```python
from build123d import *

# Parameters (mm, degrees)
SKETCH_1_W      = 150
SKETCH_1_H      = 20
SKETCH_1_W_2    = 25
SKETCH_1_H_2    = 3
EXTRUDE_1_DEPTH = 3


with BuildPart() as part:
    # 草图1 → 凸台-拉伸1 (new body)
    with BuildSketch(Plane(origin=(0, 0, 0), x_dir=(1, 0, 0), z_dir=(0, 1, 0))):
        Rectangle(SKETCH_1_W, SKETCH_1_H)
        with Locations((-60, 11.5)):
            Rectangle(SKETCH_1_W_2, SKETCH_1_H_2)
        with Locations((-60, -11.5)):
            Rectangle(SKETCH_1_W_2, SKETCH_1_H_2)
        with Locations((0, -11.5)):
            Rectangle(SKETCH_1_W_2, SKETCH_1_H_2)
        with Locations((0, 11.5)):
            Rectangle(SKETCH_1_W_2, SKETCH_1_H_2)
        with Locations((60, 11.5)):
            Rectangle(SKETCH_1_W_2, SKETCH_1_H_2)
        with Locations((60, -11.5)):
            Rectangle(SKETCH_1_W_2, SKETCH_1_H_2)
    extrude(amount=EXTRUDE_1_DEPTH)


solid = part.part
```
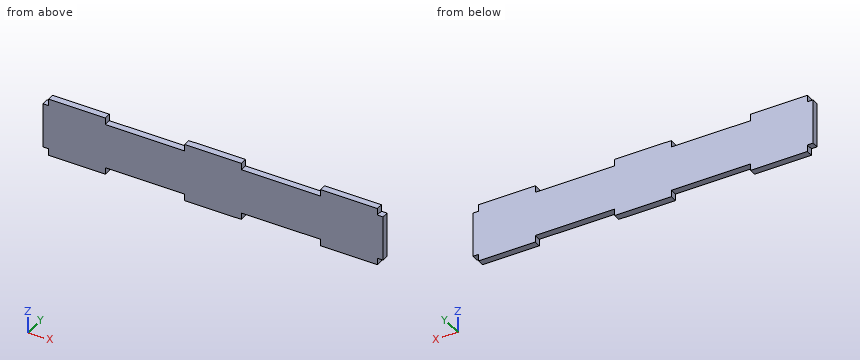
Geometry check sheet. Reference: the model listing, model coordinates, mm. Round coordinates to 2 decimals unless told otherwise and drop trailing zeros. Write each loop counter-clockwise with the first axis right and the second up, starting at its lowest first coordinate (ties: lowest second). Pieces come first, ordered by that corner, then holes. Notation, with made-up numbers: (-28.5, -18) -> (17.5, -18) arc R30 ccw to (17.5, 12) -> close; hole circle Ø7 at (71, -13.5). An arc over 180 degrees is marked (long way). Put each result on its own line as item: value.
1) Thickness scan on probe 1 along X at (y, z) = (2, 10.75); probe 2 along Z at (x, y) = (32, 1.65). Record the ranges inside material, lowest first. Write a range as from..to.
Recorded:
probe 1: x = -72.5..-47.5, -12.5..12.5, 47.5..72.5
probe 2: z = -10..10
2) Cross-section at A-A, the plane y = 0.55. Enter the section's corners in (x, z), plus the area to 3 significant figures.
Recorded:
outline: (-75, -10) -> (-72.5, -10) -> (-72.5, -13) -> (-47.5, -13) -> (-47.5, -10) -> (-12.5, -10) -> (-12.5, -13) -> (12.5, -13) -> (12.5, -10) -> (47.5, -10) -> (47.5, -13) -> (72.5, -13) -> (72.5, -10) -> (75, -10) -> (75, 10) -> (72.5, 10) -> (72.5, 13) -> (47.5, 13) -> (47.5, 10) -> (12.5, 10) -> (12.5, 13) -> (-12.5, 13) -> (-12.5, 10) -> (-47.5, 10) -> (-47.5, 13) -> (-72.5, 13) -> (-72.5, 10) -> (-75, 10) -> close
area: 3,450 mm2
3) Cross-section at B-B, the plane x = -24. Enter the section's corners in (y, z).
Recorded:
outline: (0, -10) -> (3, -10) -> (3, 10) -> (0, 10) -> close
4) Depth check by flat-ended pin: P1, Ø0.9, axis at y = 1, z = -12, coming from the -X side; P2, Ø0.9, axis at y = 1, z = -12, coming from the +X side; P3, Ø1.5, axis at x = -33, y = 2, coming from the +Z side. Enter the tip coordinate at first touch or a pass-through.
Recorded:
P1: stops at x = -72.5
P2: stops at x = 72.5
P3: stops at z = 10
